Design review of the part shown in the three views and the two pictorial views. Dimensions are in mm from the part's minimum x, y and z. Round coordinates to 2 decimals unless told otherwise and drop trailing zeros. Order: outer loops, then holes, each group sorted by start corner. A loop starts at its lowest first (then second) coordinate and runs counter-clockwise, first axis right, second up. Notation, with made-up numbers: (29.25, 35.25) -> (57.25, 35.25) arc R31 cw to (57.25, 69.25) -> close; hole circle Ø6 at (20, -34.5). An arc over 180 degrees is marked (long way). Put each result on its own line as item: value. Start each with the question number.
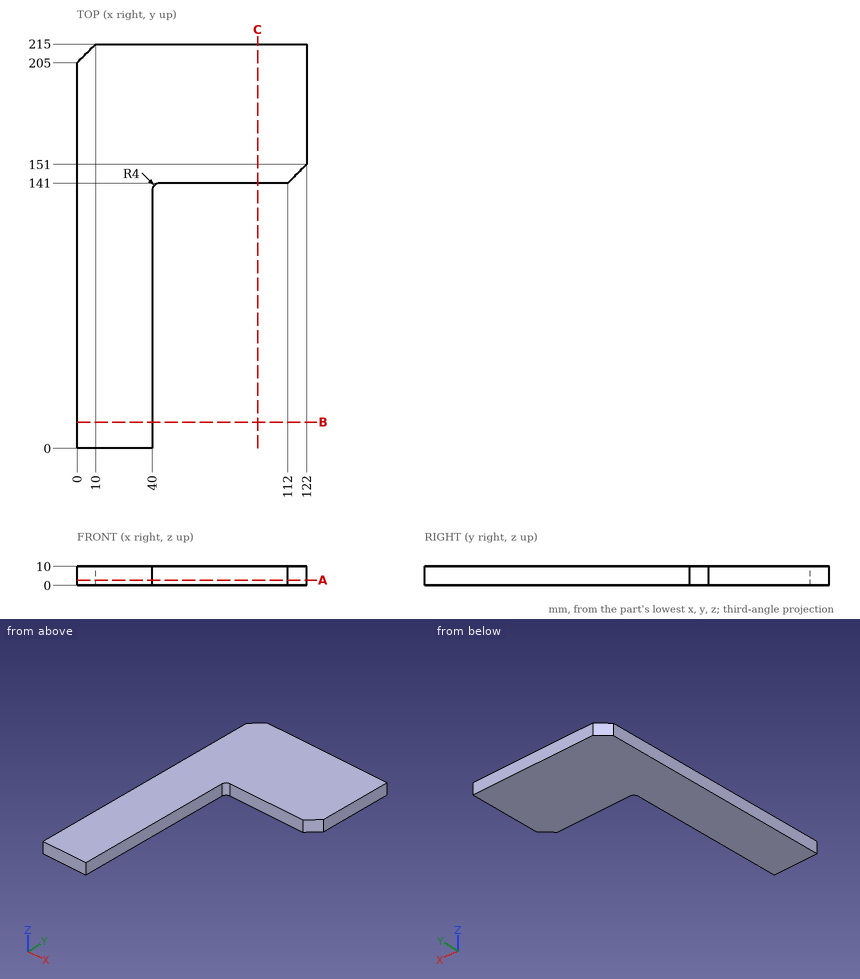
Q1. Take a section at B-B on y = 14. Give the boundary of the cut face in (x, z), and give its area (3 significant figures).
Q2. Take a section at C-C on x = 96. Give the boundary of the cut face in (y, z).
Q3. Clearance check with flat-ended pins moving along their axes: pin 1 Ø3 at (y, z) = (71.5, 4) entering from +X; pin 2 Ø1.5 at (x, z) = (58.5, 4.5) entering from -Y. State where each tip first meets the part, or that it passes through.
Q4. Wall thickness on probe 1 along X at (y, z) = (52.5, 4.25); probe 2 along Y at (x, z) = (61.5, 9); probe 3 along X at (y, z) = (149.5, 2.75): over which ranges is each line inside the solid? List them lowest first. Write a range as [from, to].
Q5. Take a section at A-A on z = 2.75. Give the boundary of the cut face in (x, y).
Calculated:
1. outline: (0, 0) -> (40, 0) -> (40, 10) -> (0, 10) -> close
1. area: 400 mm²
2. outline: (141, 0) -> (215, 0) -> (215, 10) -> (141, 10) -> close
3. pin 1: stops at x = 40
3. pin 2: stops at y = 141
4. probe 1: x = [0, 40]
4. probe 2: y = [141, 215]
4. probe 3: x = [0, 120.5]
5. outline: (0, 0) -> (40, 0) -> (40, 137) arc R4 cw to (44, 141) -> (112, 141) -> (122, 151) -> (122, 215) -> (10, 215) -> (0, 205) -> close
